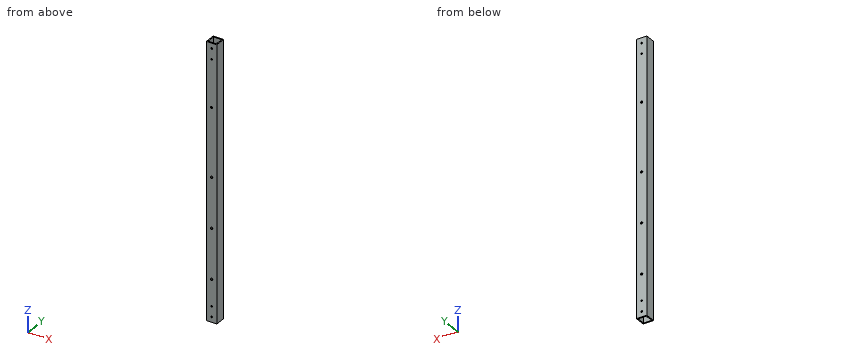
from build123d import *

# Parameters (mm, degrees)
SKETCH_1_W           = 20
SKETCH_1_H           = 20
SKETCH_1_W_2         = 16
SKETCH_1_H_2         = 16
EXTRUDE_1_DEPTH      = 560
SKETCH_4_R           = 2.2
CUT_EXTRUDE_3_DEPTH  = 560
SKETCH_5_W           = 20
SKETCH_5_H           = 20
SKETCH_5_W_2         = 16
SKETCH_5_H_2         = 16
EXTRUDE_2_DEPTH      = 20
SKETCH_6_W           = 20
SKETCH_6_H           = 20
SKETCH_6_W_2         = 16
SKETCH_6_H_2         = 16
EXTRUDE_3_DEPTH      = 20
SKETCH_8_R           = 2.2
CUT_EXTRUDE_4_DEPTH  = 20
SKETCH_9_R           = 2.2
CUT_EXTRUDE_5_DEPTH  = 20
SKETCH_10_W          = 51.42245882
SKETCH_10_H          = 30.440795882
CUT_EXTRUDE_6_DEPTH  = 40
SKETCH_11_W          = 39.362638682
SKETCH_11_H          = 52.74733359
CUT_EXTRUDE_7_DEPTH  = 40
SKETCH_12_R          = 1
CUT_EXTRUDE_8_DEPTH  = 20
SKETCH_13_R          = 1
CUT_EXTRUDE_9_DEPTH  = 20
SKETCH_15_R          = 2.2
CUT_EXTRUDE_11_DEPTH = 21
SKETCH_16_R          = 2.1
CUT_EXTRUDE_12_DEPTH = 21
M4X0_7_4_D           = 3.3
M4X0_7_5_D           = 3.3


with BuildPart() as part:
    # ｽｹｯﾁ1 → ﾎﾞｽ - 押し出し1 (new body)
    with BuildSketch(Plane.XY):
        Rectangle(SKETCH_1_W, SKETCH_1_H)
        Rectangle(SKETCH_1_W_2, SKETCH_1_H_2, mode=Mode.SUBTRACT)
    extrude(amount=EXTRUDE_1_DEPTH)

    # ｽｹｯﾁ4 → ｶｯﾄ - 押し出し3 (cut)
    with BuildSketch(Plane(origin=(0, 10, 0), x_dir=(1, 0, 0), z_dir=(0, 1, 0))):
        with Locations((0, -550)):
            Circle(SKETCH_4_R)
        with Locations((0, -10)):
            Circle(SKETCH_4_R)
    extrude(amount=-CUT_EXTRUDE_3_DEPTH, mode=Mode.SUBTRACT)

    # ｽｹｯﾁ5 → ﾎﾞｽ - 押し出し2 (add)
    with BuildSketch(Plane(origin=(0, 0, 0), x_dir=(-1, 0, 0), z_dir=(0, 0, -1))):
        Rectangle(SKETCH_5_W, SKETCH_5_H)
        Rectangle(SKETCH_5_W_2, SKETCH_5_H_2, mode=Mode.SUBTRACT)
    extrude(amount=EXTRUDE_2_DEPTH)

    # ｽｹｯﾁ6 → ﾎﾞｽ - 押し出し3 (add)
    with BuildSketch(Plane.XY.offset(560)):
        Rectangle(SKETCH_6_W, SKETCH_6_H)
        Rectangle(SKETCH_6_W_2, SKETCH_6_H_2, mode=Mode.SUBTRACT)
    extrude(amount=EXTRUDE_3_DEPTH)

    # ｽｹｯﾁ8 → ｶｯﾄ - 押し出し4 (cut)
    with BuildSketch(Plane(origin=(10, 0, 0), x_dir=(0, 0, -1), z_dir=(1, 0, 0))):
        with Locations((-570, 0)):
            Circle(SKETCH_8_R)
    extrude(amount=-CUT_EXTRUDE_4_DEPTH, mode=Mode.SUBTRACT)

    # ｽｹｯﾁ9 → ｶｯﾄ - 押し出し5 (cut)
    with BuildSketch(Plane(origin=(10, 0, 0), x_dir=(0, 0, -1), z_dir=(1, 0, 0))):
        with Locations((10, 0)):
            Circle(SKETCH_9_R)
    extrude(amount=-CUT_EXTRUDE_5_DEPTH, mode=Mode.SUBTRACT)

    # ｽｹｯﾁ10 → ｶｯﾄ - 押し出し6 (cut)
    with BuildSketch(Plane(origin=(0, 0, -20), x_dir=(-1, 0, 0), z_dir=(0, 0, -1))):
        Rectangle(SKETCH_10_W, SKETCH_10_H)
    extrude(amount=-CUT_EXTRUDE_6_DEPTH, mode=Mode.SUBTRACT)

    # ｽｹｯﾁ11 → ｶｯﾄ - 押し出し7 (cut)
    with BuildSketch(Plane.XY.offset(580)):
        Rectangle(SKETCH_11_W, SKETCH_11_H)
    extrude(amount=-CUT_EXTRUDE_7_DEPTH, mode=Mode.SUBTRACT)

    # ｽｹｯﾁ12 → ｶｯﾄ - 押し出し8 (cut)
    with BuildSketch(Plane(origin=(0, -10, 0), x_dir=(-1, 0, 0), z_dir=(0, -1, 0))):
        with Locations((0, -530)):
            Circle(SKETCH_12_R)
        with Locations((0, -510)):
            Circle(SKETCH_12_R)
    extrude(amount=-CUT_EXTRUDE_8_DEPTH, mode=Mode.SUBTRACT)

    # ｽｹｯﾁ13 → ｶｯﾄ - 押し出し9 (cut)
    with BuildSketch(Plane(origin=(0, -10, 0), x_dir=(-1, 0, 0), z_dir=(0, -1, 0))):
        with Locations((0, -30)):
            Circle(SKETCH_13_R)
        with Locations((0, -50)):
            Circle(SKETCH_13_R)
    extrude(amount=-CUT_EXTRUDE_9_DEPTH, mode=Mode.SUBTRACT)

    # ｽｹｯﾁ15 → ｶｯﾄ - 押し出し11 (cut, through all)
    with BuildSketch(Plane.XZ.offset(10)):
        with Locations((0, 100)):
            Circle(SKETCH_15_R)
        with Locations((0, 195)):
            Circle(SKETCH_15_R)
        with Locations((0, 290)):
            Circle(SKETCH_15_R)
    extrude(amount=-CUT_EXTRUDE_11_DEPTH, mode=Mode.SUBTRACT)

    # ｽｹｯﾁ16 → ｶｯﾄ - 押し出し12 (cut, through all)
    with BuildSketch(Plane.XZ.offset(10)):
        with Locations((0, 420)):
            Circle(SKETCH_16_R)
    extrude(amount=-CUT_EXTRUDE_12_DEPTH, mode=Mode.SUBTRACT)

    # M4x0.7 ねじ穴4 (through all)
    with Locations(Plane(origin=(0, -10, 30), x_dir=(0, 0, -1), z_dir=(0, -1, 0))):
        with Locations((0, 0), (-20, 0)):
            Hole(M4X0_7_4_D / 2)

    # M4x0.7 ねじ穴5 (through all)
    with Locations(Plane(origin=(0, -10, 530), x_dir=(0, 0, -1), z_dir=(0, -1, 0))):
        with Locations((0, 0), (20, 0)):
            Hole(M4X0_7_5_D / 2)


solid = part.part
Geometry: final body of the model. Coordinates: model frame, mm. Give positions to 0.01 mm unless a question says otherwise; leave off trailing zeros. Loops run counter-clockwise (first coordinate to the right, second up) from the corner with the lowest first, then second, coordinate; pieces in that order, holes last. Notation, with made-up numbers: (48, 40.25) - (96, 40.25) arc R9 cw to (96, 57.25) - close; hole circle Ø4 at (77.25, -35.5). An arc over 180 degrees is marked (long way). Answer as CSV lines item,"result". Start each with the question number.
1. Section A-A, the plane z = 69.5. Return loops of the section in (x, y), plus the area to 3 significant figures.
2. Pin query (flat end, axial travel): P1, Ø5.5, axis at x = 0, z = 30, coming from the +Y side; P2, Ø3.5, axis at x = 0, z = 420, coming from the +Y side. Return the tip coordinate at first contact, or that it passes through.
3. Ray query, L1, parallel to Y at x = -4.75, z = 283; L2, parallel to X at y = -8.6, z = 30. Return the intervals inside material, ascending.
Answers:
1,outline,"(-10, -10) - (10, -10) - (10, 10) - (-10, 10) - close; hole (-8, -8) - (8, -8) - (8, 8) - (-8, 8) - close"
1,area,"144 mm2"
2,P1,"stops at y = 10"
2,P2,"passes through"
3,L1,"y = -10 to -8, 8 to 10"
3,L2,"x = -10 to -1.65, 1.65 to 10"
